```python
from build123d import *

# Parameters (mm, degrees)
BOSS_EXTRU_1_DEPTH      = 15
ESQUISSE2_R             = 1.5
ENL_V_MAT_EXTRU_1_DEPTH = 5
ESQUISSE3_R             = 1.5
ENL_V_MAT_EXTRU_2_DEPTH = 5


with BuildPart() as part:
    # Esquisse1 → Boss.-Extru.1 (new body)
    with BuildSketch(Plane.XY):
        Polygon((0, -3.464101615), (3, -1.732050808), (3, 1.732050808), (0, 3.464101615), (-3, 1.732050808), (-3, -1.732050808), align=None)
    extrude(amount=BOSS_EXTRU_1_DEPTH)

    # Esquisse2 → Enlèv. mat.-Extru.1 (cut)
    with BuildSketch(Plane(origin=(0, 0, 0), x_dir=(-1, 0, 0), z_dir=(0, 0, -1))):
        Circle(ESQUISSE2_R)
    extrude(amount=-ENL_V_MAT_EXTRU_1_DEPTH, mode=Mode.SUBTRACT)

    # Esquisse3 → Enlèv. mat.-Extru.2 (cut)
    with BuildSketch(Plane.XY.offset(15)):
        Circle(ESQUISSE3_R)
    extrude(amount=-ENL_V_MAT_EXTRU_2_DEPTH, mode=Mode.SUBTRACT)


solid = part.part
```
CAD build for the part. Positions are in the model's coordinates, mm. A direction names the side the tool comes from. Round coordinates to 2 decimals unless told otherwise and drop trailing zeros. Loops run counter-clockwise (first coordinate to the right, second up) from the corner with the lowest first, then second, coordinate; pieces in that order, holes last. Notation, with made-up numbers: M 66.25,67 L 78.25,67 A12 ccw 78.25,86 Z; hole C 69,44 d4. An arc over 180 degrees is marked long. Use a Markdown table: item, result. Add a question column.
(1) Cut at A-A (z = 12.75). Give the cut face in (x, y).
(2) Cut at C-C (z = 8.75). Give the cut face in (x, y), and give its area (3 significant figures).
(3) Pull direction X, two halves, no side cores. Call faces 4 (the face through (1.5, 2.6, 7.4)), 5 (the face through (-3, 0, 7)), 6 (the face through (0, 0, 5)), 7 (the face through (-1.5, 0.07, 12.54)): +X half, -X half, draft (parallel to the pull), parting line (faces both ways), or undercut.
(4) Flat gauge pins, fed straight in: pin 1 (1.5 mm diameter, centred on x = 1, z = 7.5, fed in from +Y); pin 2 (1.5 mm diameter, centred on x = 1, z = 9.5, fed in from -Y); pin 3 (1.8 mm diameter, centred on x = 0, y = 0, fed in from -Z). Where does each tip first touch, or does it go through?
(5) Which spindle directions (+Z, -Z, +X, -X, +Y, -Y) get a long thin tool onto all of the face, cutting with end or side? Do faces 1 (the face through (1.5, 0.07, 2.46)), 2 (the face through (3, 0, 7)), 3 (the face through (0, 0, 10)). Say none if no direction does.
(6) Drill centre lines: line 1 (X direction, y = -1, z = 13.25); line 2 (X direction, y = -0.5, z = 12.75); line 3 (Y direction, x = 0.5, z = 4.5). Where is each one in solid material? Low to high.
(7) Cut at B-B (y = 0). Give the cut face in (x, z), and give its area (3 significant figures).
(8) Cut at D-D (x = -0.25). Give the cut face in (y, z), and give its area (3 significant figures).
Geometry says:
| question | item | result |
|---|---|---|
| 1 | outline | M -3,-1.73 L 0,-3.46 L 3,-1.73 L 3,1.73 L 0,3.46 L -3,1.73 Z; hole C 0,0 d3 |
| 2 | outline | M -3,-1.73 L 0,-3.46 L 3,-1.73 L 3,1.73 L 0,3.46 L -3,1.73 Z |
| 2 | area | 31.2 mm² |
| 3 | face 4 | +X half |
| 3 | face 5 | -X half |
| 3 | face 6 | undercut |
| 3 | face 7 | undercut |
| 4 | pin 1 | stops at y = 3.32 |
| 4 | pin 2 | stops at y = -3.32 |
| 4 | pin 3 | stops at z = 5 |
| 5 | face 1 | -Z |
| 5 | face 2 | +Z, -Z, +X, +Y, -Y |
| 5 | face 3 | +Z |
| 6 | line 1 | x = -3 to -1.12, 1.12 to 3 |
| 6 | line 2 | x = -3 to -1.41, 1.41 to 3 |
| 6 | line 3 | y = -3.18 to -1.41, 1.41 to 3.18 |
| 7 | outline | M -3,0 L -1.5,0 L -1.5,5 L 1.5,5 L 1.5,0 L 3,0 L 3,15 L 1.5,15 L 1.5,10 L -1.5,10 L -1.5,15 L -3,15 Z |
| 7 | area | 60.0 mm² |
| 8 | outline | M -3.32,0 L -1.48,0 L -1.48,5 L 1.48,5 L 1.48,0 L 3.32,0 L 3.32,15 L 1.48,15 L 1.48,10 L -1.48,10 L -1.48,15 L -3.32,15 Z |
| 8 | area | 70.0 mm² |
